```python
from build123d import *

# Parameters (mm, degrees)
BOSS_EXTRUDE1_DEPTH      = 2
BOSS_EXTRUDE1_DEPTH_BACK = 2
BOSS_EXTRUDE2_DEPTH      = 2
CUT_EXTRUDE2_DEPTH       = 3
BOSS_EXTRUDE3_DEPTH      = 3
BOSS_EXTRUDE3_DEPTH_BACK = 4
BOSS_EXTRUDE4_DEPTH      = 5.768626
BOSS_EXTRUDE5_DEPTH      = 7
CUT_EXTRUDE3_DEPTH       = 106.532768689


with BuildPart() as part:
    # Sketch1 → Boss-Extrude1 (new body, two sides)
    with BuildSketch(Plane.XY) as boss_extrude1_sk:
        with BuildLine():
            ThreePointArc((-99.883719426, -303.368163267), (-118.083910473, -292.687102225), (-129.239344224, -274.773746399))
            Line((-129.239344224, -274.773746399), (-122.900985764, -246.890150727))
            ThreePointArc((-122.900985764, -246.890150727), (-126.803064599, -240.933983923), (-126.548538034, -233.817990776))
            Line((-126.548538034, -233.817990776), (-119.123281802, -208.687862835))
            ThreePointArc((-119.123281802, -208.687862835), (-107.698999343, -197.140529866), (-92.168900704, -192.379105219))
            Line((-92.168900704, -192.379105219), (-64.113961972, -192.379105219))
            ThreePointArc((-64.113961972, -192.379105219), (-31.572672129, -197.617974675), (-3.509282377, -214.904601108))
            ThreePointArc((-3.509282377, -214.904601108), (-3.309447715, -231.856766436), (-15.259350681, -243.882391671))
            Line((-15.259350681, -243.882391671), (-13.742027997, -259.699185691))
            ThreePointArc((-13.742027997, -259.699185691), (-20.907511644, -286.149918063), (-42.397436123, -303.15487454))
            ThreePointArc((-42.397436123, -303.15487454), (-63.833611273, -306.582364975), (-85.533592749, -305.975652807))
            Line((-85.533592749, -305.975652807), (-99.883719426, -303.368163267))
        make_face()
        with BuildLine():
            add(Edge.make_bspline(
                [(-17.415513131, -242.668556981), (-16.250894512, -241.965818827), (-15.109288702, -241.224994889), (-13.441213679, -240.040387525), (-12.89262097, -239.633218083), (-11.812693685, -238.790317301), (-11.280400788, -238.353703672), (-9.726955108, -237.00465557), (-8.745390801, -236.051712079), (-7.385039015, -234.511313148), (-6.948715528, -233.976815867), (-6.130845571, -232.874503238), (-5.750270787, -232.30842269), (-4.706493232, -230.558637643), (-4.138677409, -229.324736835), (-3.562547958, -227.328857227), (-3.422001152, -226.654431705), (-3.252657323, -225.296308422), (-3.223357134, -224.611043663), (-3.269242402, -223.573082537), (-3.29957286, -223.227633129), (-3.388711058, -222.546593141), (-3.476993493, -222.041163228), (-3.596272382, -221.543472132), (-3.682574516, -221.213371534), (-3.730157677, -221.049427786), (-4.247949017, -219.244642568), (-4.718668417, -217.603928734), (-5.189387817, -215.9632149)],
                knots=[0, 0, 0, 0, 0.125, 0.125, 0.1875, 0.1875, 0.25, 0.25, 0.375, 0.375, 0.4375, 0.4375, 0.5, 0.5, 0.625, 0.625, 0.6875, 0.6875, 0.75, 0.75, 0.78125, 0.78125, 0.8125, 0.828125, 0.828125, 0.84375, 0.84375, 1, 1, 1, 1], degree=3))
            ThreePointArc((-5.189387817, -215.9632149), (-32.526455477, -199.407751302), (-64.08963442, -194.391340409))
            Line((-64.08963442, -194.391340409), (-92.144573152, -194.392657625))
            Line((-92.144573152, -194.392657625), (-92.202629041, -194.392657625))
            ThreePointArc((-92.202629041, -194.392657625), (-106.647929369, -198.873907617), (-117.312202813, -209.598718803))
            Line((-117.312202813, -209.598718803), (-124.435145464, -234.429494019))
            ThreePointArc((-124.435145464, -234.429494019), (-124.604366095, -241.045289532), (-120.469878975, -246.212823))
            Line((-120.469878975, -246.212823), (-121.332617267, -249.132685018))
            Line((-121.332617267, -249.132685018), (-127.264768762, -275.229302117))
            ThreePointArc((-127.264768762, -275.229302117), (-116.098302818, -291.621676712), (-98.954802842, -301.596661178))
            ThreePointArc((-98.954802842, -301.596661178), (-70.952790665, -304.90715996), (-42.984896901, -301.319820198))
            ThreePointArc((-42.984896901, -301.319820198), (-22.606132147, -285.170975908), (-15.696872441, -260.104237885))
            Line((-15.696872441, -260.104237885), (-17.415513131, -242.668556981))
        make_face(mode=Mode.SUBTRACT)
    extrude(amount=BOSS_EXTRUDE1_DEPTH)
    extrude(boss_extrude1_sk.sketch, amount=-BOSS_EXTRUDE1_DEPTH_BACK)

    # Sketch4 → Boss-Extrude2 (add)
    with BuildSketch(Plane.XY.offset(2)):
        with BuildLine():
            Line((-121.332617267, -249.132685018), (-127.264768762, -275.229302117))
            ThreePointArc((-127.264768762, -275.229302117), (-116.098302818, -291.621676712), (-98.954802842, -301.596661178))
            ThreePointArc((-98.954802842, -301.596661178), (-70.952790665, -304.90715996), (-42.984896901, -301.319820198))
            ThreePointArc((-42.984896901, -301.319820198), (-22.606132147, -285.170975908), (-15.696872441, -260.104237885))
            Line((-15.696872441, -260.104237885), (-17.415513131, -242.668556981))
            add(Edge.make_bspline(
                [(-17.415513131, -242.668556981), (-16.250894512, -241.965818827), (-15.109288702, -241.224994889), (-13.441213679, -240.040387525), (-12.89262097, -239.633218083), (-11.812693685, -238.790317301), (-11.280400788, -238.353703672), (-9.726955108, -237.00465557), (-8.745390801, -236.051712079), (-7.385039015, -234.511313148), (-6.948715528, -233.976815867), (-6.130845571, -232.874503238), (-5.750270787, -232.30842269), (-4.706493232, -230.558637643), (-4.138677409, -229.324736835), (-3.562547958, -227.328857227), (-3.422001152, -226.654431705), (-3.252657323, -225.296308422), (-3.223357134, -224.611043663), (-3.269242402, -223.573082537), (-3.29957286, -223.227633129), (-3.388711058, -222.546593141), (-3.476993493, -222.041163228), (-3.596272382, -221.543472132), (-3.682574516, -221.213371534), (-3.730157677, -221.049427786), (-4.247949017, -219.244642568), (-4.718668417, -217.603928734), (-5.189387817, -215.9632149)],
                knots=[0, 0, 0, 0, 0.125, 0.125, 0.1875, 0.1875, 0.25, 0.25, 0.375, 0.375, 0.4375, 0.4375, 0.5, 0.5, 0.625, 0.625, 0.6875, 0.6875, 0.75, 0.75, 0.78125, 0.78125, 0.8125, 0.828125, 0.828125, 0.84375, 0.84375, 1, 1, 1, 1], degree=3))
            ThreePointArc((-5.189387817, -215.9632149), (-32.526455477, -199.407751302), (-64.08963442, -194.391340409))
            Line((-64.08963442, -194.391340409), (-92.144573152, -194.392657625))
            Line((-92.144573152, -194.392657625), (-92.202629041, -194.392657625))
            ThreePointArc((-92.202629041, -194.392657625), (-106.647929369, -198.873907617), (-117.312202813, -209.598718803))
            Line((-117.312202813, -209.598718803), (-124.435145464, -234.429494019))
            ThreePointArc((-124.435145464, -234.429494019), (-124.604366095, -241.045289532), (-120.469878975, -246.212823))
            Line((-120.469878975, -246.212823), (-121.332617267, -249.132685018))
        make_face()
    extrude(amount=-BOSS_EXTRUDE2_DEPTH)

    # Sketch5 → Cut-Extrude2 (cut)
    with BuildSketch(Plane(origin=(0.009126788, -194.388330888, 0), x_dir=(0.999999999, 4.6951e-05, 0), z_dir=(4.6951e-05, -0.999999999, 0))):
        Polygon((-92.153700041, 0), (-92.21175593, 0), (-92.21175593, -2), (-92.153700041, -2), (-64.098761279, -2), (-64.098761279, 0), align=None)
    extrude(amount=-CUT_EXTRUDE2_DEPTH, mode=Mode.SUBTRACT)

    # Sketch6 → Boss-Extrude3 (add, two sides)
    with BuildSketch(Plane(origin=(0, 0, -2), x_dir=(-1, 0, 0), z_dir=(0, 0, -1))) as boss_extrude3_sk:
        with BuildLine():
            Line((10.862265169, -211.246797097), (9.680301702, -209.700960004))
            Line((9.680301702, -209.700960004), (14.382573251, -206.353642546))
            Line((14.382573251, -206.353642546), (15.461710653, -207.995655709))
            ThreePointArc((15.461710653, -207.995655709), (13.134440717, -209.582254915), (10.862265169, -211.246797097))
        make_face()
    extrude(amount=BOSS_EXTRUDE3_DEPTH)
    extrude(boss_extrude3_sk.sketch, amount=-BOSS_EXTRUDE3_DEPTH_BACK)



with BuildPart() as body_2:
    # Sketch7 → Boss-Extrude4 (new body)
    with BuildSketch(Plane(origin=(95.075403567, -72.695663841, 0), x_dir=(0, 0, -1), z_dir=(0.794394345, -0.607402358, 0))):
        with BuildLine():
            Line((-2, -172.465094912), (5, -172.465094912))
            ThreePointArc((5, -172.465094912), (2.949747468, -167.515347444), (-2, -165.465094912))
            Line((-2, -165.465094912), (-2, -172.465094912))
        make_face()
    extrude(amount=-BOSS_EXTRUDE4_DEPTH)


with BuildPart() as part_1:
    add(part.part)

    add(body_2.part)  # Boss-Extrude5 merges body 2
    # Sketch8 → Boss-Extrude5 (add)
    with BuildSketch(Plane(origin=(0, 0, -5), x_dir=(-1, 0, 0), z_dir=(0, 0, -1))):
        Polygon((14.26286593, -206.197082701), (14.382573251, -206.353642546), (9.680301702, -209.700960004), align=None)
    extrude(amount=-BOSS_EXTRUDE5_DEPTH)

    # Sketch9 → Cut-Extrude3 (cut, through all)
    with BuildSketch(Plane(origin=(95.075403567, -72.695663841, 0), x_dir=(0, 0, -1), z_dir=(0.794394345, -0.607402358, 0))):
        Polygon((-2, -165.465094912), (5, -174.411026553), (7.216406638, -174.411026553), (7.216406638, -165.465094912), align=None)
    extrude(amount=-CUT_EXTRUDE3_DEPTH, mode=Mode.SUBTRACT)


solid = part_1.part
```
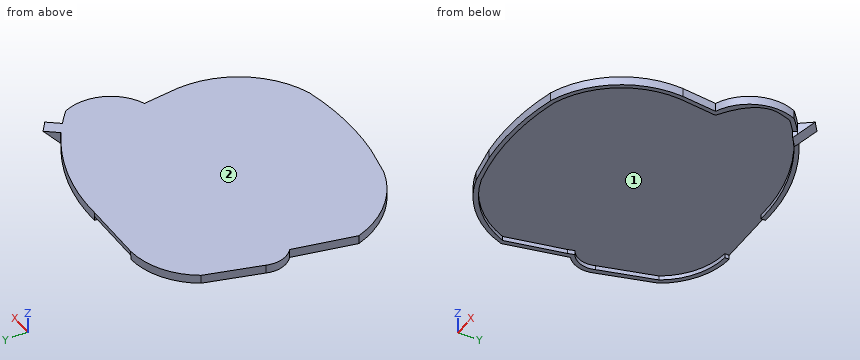
Source: CAD feature listing. Evaluate the final solid. Frame: model axes, mm. Face numbers are marked on the shaded views. Round coordinates to 2 decimals unless told otherwise and drop trailing zeros. Loops run counter-clockwise (first coordinate to the right, second up) from the corner with the lowest first, then second, coordinate; pieces in that order, holes last. Notation, with made-up numbers: M -32,52 L 3,52 A27 ccw 3,71 Z; hole C -30.5,26.25 d1. An arc over 180 degrees is marked long. Use a Markdown table: item, result. Add a question column.
1. Ray query, line 1 along Z through (x, y) = (-103.5, -243); line 2 along Z through (x, y) = (-109, -199); line 3 along X through (y, z) = (-234.5, -0.25). Return the intervals inside material, ascending. Write a range as [from, to].
2. Contact query for flat-ended pins moving along their axis: pin 1 (1.5 mm diameter, centred on y = -211, z = 0.5, fed in from +X); pin 2 (8 mm diameter, centred on x = -26.5, y = -250.5, fed in from -Z); pin 3 (1 mm diameter, centred on y = -252.5, z = -3.5, fed in from -X); pin 4 (3 mm diameter, centred on y = -292.5, z = -2, fed in from +X). Output: stop coordinate, or through.
3. Cut plane B-B, the plane x = -27. Output: boundary loops of the cut face in (y, z).
4. Pull-direction query (Y, two-part tool) for the marked faces 1 and 2; classes: +Y half, -Y half, draft (parallel to the pull), parting line (faces both ways), or undercut.
5. Cut plane C-C, the plane x = -67.5. Output: boundary loops of the cut face in (y, z).
6. Cut plane A-A, the plane y = -261.5. Output: boundary loops of the cut face in (x, z), and give its area (3 significant figures).
Solution:
| question | item | result |
|---|---|---|
| 1 | line 1 | z = [0, 2] |
| 1 | line 2 | z = [-2, 2] |
| 1 | line 3 | x = [-126.77, -124.46], [-7.39, -4.59] |
| 2 | pin 1 | stops at x = -7.11 |
| 2 | pin 2 | stops at z = 0 |
| 2 | pin 3 | passes through |
| 2 | pin 4 | stops at x = -24.62 |
| 3 | outline | M -293.5,-2 L -290.72,-2 L -290.72,0 L -201.66,0 L -201.66,-2 L -199.47,-2 L -199.47,2 L -293.5,2 Z |
| 4 | face 1 | undercut |
| 4 | face 2 | draft |
| 5 | outline | M -306.76,-2 L -304.84,-2 L -304.84,0 L -192.38,0 L -192.38,2 L -306.76,2 Z |
| 6 | outline | M -126.22,-2 L -124.14,-2 L -124.14,0 L -15.65,0 L -15.65,-2 L -13.68,-2 L -13.68,2 L -126.22,2 Z |
| 6 | area | 233 mm2 |
